from build123d import *

# Parameters (mm, degrees)
SKETCH_1_W      = 35
SKETCH_1_H      = 10
SKETCH_1_R      = 2.1
EXTRUDE_1_DEPTH = 2.5
SKETCH_3_R      = 1.6
EXTRUDE_2_DEPTH = 2.5
EXTRUDE_3_DEPTH = 2.5
FILLET_1_R      = 2


with BuildPart() as part:
    # 草图1 → 凸台-拉伸1 (new body)
    with BuildSketch(Plane(origin=(0, 0, 0), x_dir=(1, 0, 0), z_dir=(0, 1, 0))):
        Rectangle(SKETCH_1_W, SKETCH_1_H)
        with Locations(Location((-7.5, 0, 0), (0, 0, 270))):
            Circle(SKETCH_1_R, mode=Mode.SUBTRACT)
        with Locations(Location((7.5, 0, 0), (0, 0, 270))):
            Circle(SKETCH_1_R, mode=Mode.SUBTRACT)
    extrude(amount=EXTRUDE_1_DEPTH)

    # 草图3 → 凸台-拉伸2 (add)
    with BuildSketch(Plane(origin=(0, 2.5, 0), x_dir=(1, 0, 0), z_dir=(0, 1, 0))):
        Polygon((-17.5, -5), (17.5, -5), (17.5, -50.601870189), (-17.5, -46.304410557), align=None)
        with Locations(Location((-10, -17, 0), (0, 0, 270))):
            Circle(SKETCH_3_R, mode=Mode.SUBTRACT)
        with Locations(Location((9.850923033, -19.437386868, 0), (0, 0, 270))):
            Circle(SKETCH_3_R, mode=Mode.SUBTRACT)
    extrude(amount=-EXTRUDE_2_DEPTH)

    # 草图4 → 凸台-拉伸3 (add)
    with BuildSketch(Plane(origin=(0, 2.5, 0), x_dir=(1, 0, 0), z_dir=(0, 1, 0))):
        Polygon((21.083035005, -51.041811568), (27.808689923, 3.734252034), (17.5, 5), (17.5, -50.601870189), align=None)
    extrude(amount=-EXTRUDE_3_DEPTH)

    # 圆角1
    fillet_1_edges = [part.edges().sort_by_distance(p)[0] for p in [
        (-17.5, 1.25, 46.304410557),
        (21.083035005, 1.25, 51.041811568),
        (27.808689923, 1.25, -3.734252034),
        (-17.5, 1.25, -5),
        (17.5, 1.25, -5),
    ]]
    fillet(fillet_1_edges, radius=FILLET_1_R)


solid = part.part
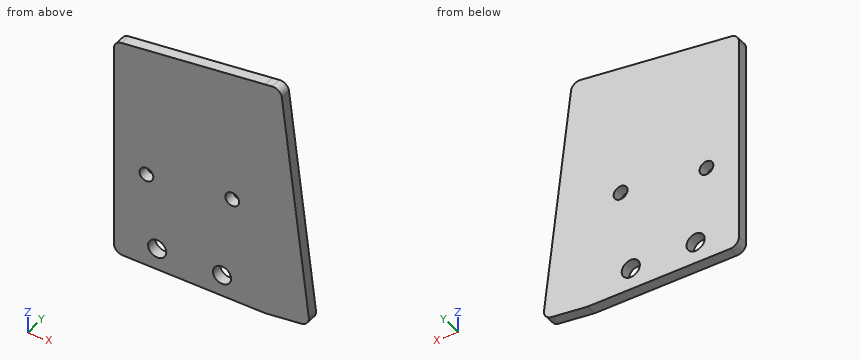
Verification items for the finished model (mm, model axes). Coordinates: 2 decimals unless noted, no trailing zeros. Loops run counter-clockwise (first coordinate to the right, second up) from the corner with the lowest first, then second, coordinate; pieces in that order, holes last. Notation, with made-up numbers: (-36.75, -10) -> (-25.75, -10) arc R17 cw to (-25.75, 5) -> close; hole circle Ø6 at (30, -17). An arc over 180 degrees is marked (long way). Answer as a JSON object with one key per item and string values. Group by question number.
Item 1: Sectioned sample at A-A on z = 17. Record the boundary of the cut face in (x, y).
Item 2: Depth check by flat-ended pin: pin 1 (1.9 mm diameter, centred on x = -10, z = 17, fed in from -Y); pin 2 (1.5 mm diameter, centred on y = 0.5, z = 12.5, fed in from +X). Enter the tip coordinate at first touch or a pass-through.
Item 3: Sectioned sample at C-C on x = 7.5. Record the boundary of the cut face in (y, z), plus the area to 3 significant figures.
Item 4: Sectioned sample at B-B on y = 0.9. Record the boundary of the cut face in (x, z).
Item 5: Scan lines: probe 1 along X at (y, z) = (0.25, 0); probe 2 along X at (y, z) = (1.7, 16); probe 3 along X at (y, z) = (1.65, 20). Record each from-to range of solid material in increasing order.
Item 6: Sectioned sample at D-D on z = 0. Record the boundary of the cut face in (x, y).
Evaluation:
{
 "1": {"outline": "(-17.5, 0) -> (-11.6, 0) -> (-11.6, 2.5) -> (-17.5, 2.5) -> close; (-8.4, 0) -> (25.26, 0) -> (25.26, 2.5) -> (-8.4, 2.5) -> close"},
 "2": {"pin 1": "passes through", "pin 2": "stops at x = 25.91"},
 "3": {"outline": "(0, -5) -> (2.5, -5) -> (2.5, -2.1) -> (0, -2.1) -> close; (0, 2.1) -> (2.5, 2.1) -> (2.5, 49.37) -> (0, 49.37) -> close", "area": "125 mm²"},
 "4": {"outline": "(-17.5, -3) arc R2 ccw to (-15.5, -5) -> (17.38, -5) arc R2 ccw to (17.62, -4.99) -> (25.82, -3.98) arc R2 ccw to (27.56, -1.75) -> (21.33, 49.06) arc R2 ccw to (19.1, 50.8) -> (-15.74, 46.52) arc R2 ccw to (-17.5, 44.53) -> close; hole circle Ø3.2 at (-10, 17); hole circle Ø4.2 at (-7.5, 0); hole circle Ø4.2 at (7.5, 0); hole circle Ø3.2 at (9.85, 19.44)"},
 "5": {"probe 1": "x = -17.5 to -9.6, -5.4 to 5.4, 9.6 to 27.35", "probe 2": "x = -17.5 to -11.25, -8.75 to 25.39", "probe 3": "x = -17.5 to 8.35, 11.35 to 24.89"},
 "6": {"outline": "(-17.5, 0) -> (-9.6, 0) -> (-9.6, 2.5) -> (-17.5, 2.5) -> close; (-5.4, 0) -> (5.4, 0) -> (5.4, 2.5) -> (-5.4, 2.5) -> close; (9.6, 0) -> (27.35, 0) -> (27.35, 2.5) -> (9.6, 2.5) -> close"}
}
